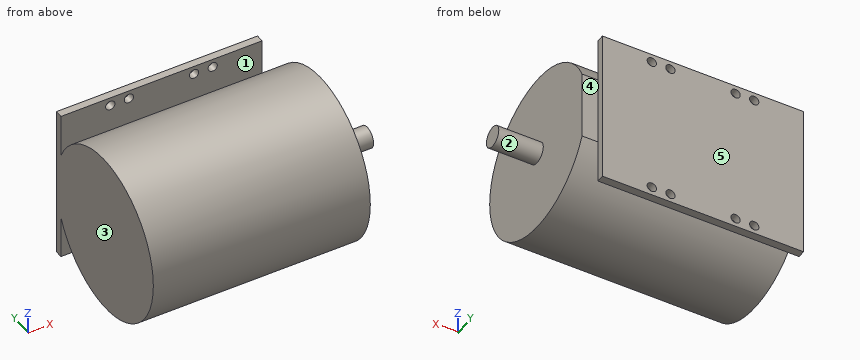
```python
from build123d import *

# Parameters (mm, degrees)
F0_W          = 274.32
F0_H          = 213.36
F0_R          = 6.35
F1_DEPTH      = 10.414
F3_DEPTH      = 21.59
F3_DEPTH_BACK = 274.32
F4_R          = 14.2875
F5_DEPTH      = 60.706


with BuildPart() as f1:
    # F0 (on Front) → F1 (new body)
    with BuildSketch(Plane.XZ):
        with Locations((-81.1550752527, 15.3063097969)):
            Rectangle(F0_W, F0_H)
        with Locations((-151.0050752527, -79.9436902031)):
            Circle(F0_R, mode=Mode.SUBTRACT)
        with Locations((-125.6050752527, -79.9436902031)):
            Circle(F0_R, mode=Mode.SUBTRACT)
        with Locations((-36.7050752527, -79.9436902031)):
            Circle(F0_R, mode=Mode.SUBTRACT)
        with Locations((-11.3050752527, -79.9436902031)):
            Circle(F0_R, mode=Mode.SUBTRACT)
        with Locations((-151.0050752527, 110.5563097969)):
            Circle(F0_R, mode=Mode.SUBTRACT)
        with Locations((-125.6050752527, 110.5563097969)):
            Circle(F0_R, mode=Mode.SUBTRACT)
        with Locations((-36.7050752527, 110.5563097969)):
            Circle(F0_R, mode=Mode.SUBTRACT)
        with Locations((-11.3050752527, 110.5563097969)):
            Circle(F0_R, mode=Mode.SUBTRACT)
    extrude(amount=F1_DEPTH)

    # F2 (on face) → F3 (join, two sides)
    with BuildSketch(Plane.YZ.offset(56.0049247473)) as f3_sk:
        with BuildLine():
            Line((-10.414, -31.8310537272), (-10.414, 62.4436733209))
            ThreePointArc((-10.414, 62.4436733209), (-223.774, 15.3063097969), (-10.414, -31.8310537272))
        make_face()
    extrude(amount=F3_DEPTH)
    extrude(f3_sk.sketch, amount=-F3_DEPTH_BACK)

    # F4 (on face) → F5 (join)
    with BuildSketch(Plane.YZ.offset(77.5949247473)):
        with Locations((-114.3, 15.3063097969)):
            Circle(F4_R)
    extrude(amount=F5_DEPTH)


solid = f1.part
```
Work out the finished part from the listing and answer in its coordinate system (mm). Face numbers are marked on the shaded views. A direction names the side the tool comes from. Give positions to 0.01 mm unless a question says otherwise; leave off trailing zeros. Loops run counter-clockwise (first coordinate to the right, second up) from the corner with the lowest first, then second, coordinate; pieces in that order, holes last. Notation, with made-up numbers: (53.25, 52.5) -> (99.25, 52.5) arc R27 cw to (99.25, 86.5) -> close; hole circle Ø2 at (71, 24.25). An arc over 180 degrees is marked (long way). Put each result on its own line as item: value. Start each with the question number.
Item 1: Find the intervals of material crossed by L1, parallel to X at y = -48, z = -34; L2, parallel to Y at x = -25, z = -61; L3, parallel to Y at x = -149.5, z = -86.5, in increasing order. Write a range as [from, to].
Item 2: The mould has two halves that part along Y. Classify the marked faces 1, 2 and 3: released by +Y, released by -Y, zero draft, split by the parting line, or undercut.
Item 3: Each of these flat-tipped pins is pushed along its axis until it touches: P1, Ø5, axis at x = -129, z = -36, coming from the -Y side; P2, Ø4, axis at x = -138.5, z = 0.5, coming from the -Y side; P3, Ø16.5, axis at x = -125.61, z = -79.94, coming from the -Y side. Where does it stop, or does it pass through?
Item 4: The part is cut by section B-B (y = -114.3). Give the vertices of the cut face in (x, z).
Item 5: The part is cut by section A-A (z = -45). Give the vertices of the cut face in (x, y), then the cut area to 3 significant figures.
Item 6: The part is cut by section C-C (x = -175). Give the vertices of the cut face in (y, z).
Item 7: The part is cut by section D-D (z = 25.5). Give the vertices of the cut face in (x, y), then the cut area to 3 significant figures.
Item 8: Which of the six approach directions +Z, -Z, +X, -X, +Y, -Y give full straight-line access (tool end or side, diameter ignored) to the marked faces 4 and 5?
Answers below:
1. L1: [-218.32, 77.59]
1. L2: [-193.72, -30.06], [-10.41, 0]
1. L3: [-158.3, -65.47], [-10.41, 0]
2. face 1: undercut
2. face 2: split by the parting line
2. face 3: zero draft
3. P1: y = -212.57
3. P2: y = -223.04
3. P3: y = -182.25
4. outline: (-218.32, -96.55) -> (77.59, -96.55) -> (77.59, 1.02) -> (138.3, 1.02) -> (138.3, 29.59) -> (77.59, 29.59) -> (77.59, 127.17) -> (-218.32, 127.17) -> close
5. outline: (-218.32, -206.13) -> (77.59, -206.13) -> (77.59, -17.64) -> (-218.32, -17.64) -> close; (-218.32, -10.41) -> (56, -10.41) -> (56, 0) -> (-218.32, 0) -> close
5. area: 58,600 mm2
6. outline: (-10.41, -91.37) -> (0, -91.37) -> (0, 121.99) -> (-10.41, 121.99) -> (-10.41, 62.44) arc R111.89 ccw (long way) to (-10.41, -31.83) -> close
7. outline: (-218.32, -223.31) -> (77.59, -223.31) -> (77.59, -124.31) -> (138.3, -124.31) -> (138.3, -104.29) -> (77.59, -104.29) -> (77.59, -10.41) -> (56, -10.41) -> (56, 0) -> (-218.32, 0) -> close
7. area: 67,100 mm2
8. face 4: +Z, -Z, +X, +Y
8. face 5: +Z, -Z, +X, -X, +Y
